Part model, mm, in its own coordinate system. Face numbers are marked on the shaded views. Coordinates: 2 decimals unless noted, no trailing zeros. Write each loop counter-clockwise with the first axis right and the second up, starting at its lowest first coordinate (ties: lowest second). Pieces come first, ordered by that corner, then holes. Notation, with made-up numbers: M 74.5,-3.75 L 114.5,-3.75 A16 ccw 114.5,10.25 Z; hole C -38,73 d10. An arc over 180 degrees is marked long. Use a Markdown table: item, result. Add a question column.
Q1. Slice it at B-B on y = 0. Write the cut outline in (x, z), then the cut area to 3 significant figures.
Q2. Slice it at D-D on z = 5.5. Write the cut outline in (x, y).
Q3. Wall check: L1, parallel to Y at x = -34, z = 3.5; L2, parallel to Y at x = -12.5, z = 5.25; L3, parallel to X at y = -29, z = 2. Give the ranges that are in metal, low to high. Write a range as from..to.
Q4. Mould opens along Y. For the marked faces 1, 2 and 3 say: released by +Y, released by -Y, zero draft, split by the parting line, or undercut.
Q5. Slice it at C-C on x = 50.5. Write the cut outline in (y, z).
Q6. Pin check, flat tips, straight feed: pin 1 Ø3 at (x, z) = (-56.5, 5.5) entering from +Y; pin 2 Ø3 at (y, z) = (-53, 3.5) entering from -X; pin 3 Ø5 at (x, z) = (25.5, 2) entering from +Y. Stop position of each tip, or through.
Q7. Slice it at A-A on x = 0. Write the cut outline in (y, z).
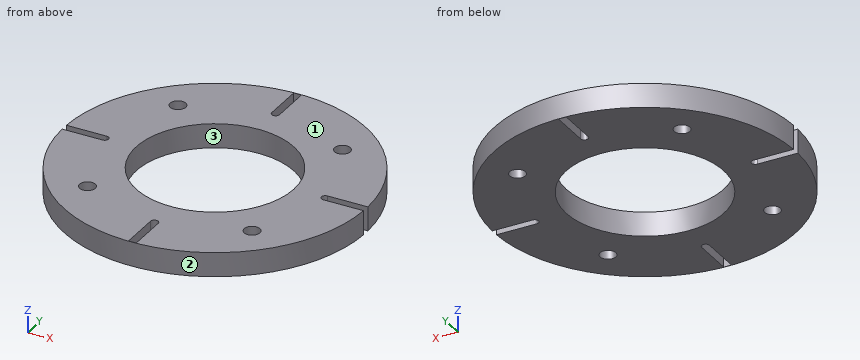
from build123d import *

# Parameters (mm, degrees)
IZIM1_R                     = 62.2
Y_KSEKLIK_EKSTR_ZYON1_DEPTH = 10
IZIM2_R                     = 32.5
KES_EKSTR_ZYON1_DEPTH       = 10
KES_EKSTR_ZYON2_DEPTH       = 10
IZIM5_R                     = 3.25
KES_EKSTR_ZYON3_DEPTH       = 10


with BuildPart() as part:
    # Çizim1 → Yükseklik-Ekstrüzyon1 (new body)
    with BuildSketch(Plane.XY):
        Circle(IZIM1_R)
    extrude(amount=Y_KSEKLIK_EKSTR_ZYON1_DEPTH)

    # Çizim2 → Kes-Ekstrüzyon1 (cut)
    with BuildSketch(Plane.XY.offset(10)):
        Circle(IZIM2_R)
    extrude(amount=-KES_EKSTR_ZYON1_DEPTH, mode=Mode.SUBTRACT)

    # Çizim4 → Kes-Ekstrüzyon2 (cut)
    with BuildSketch(Plane.XY.offset(10)):
        with BuildLine():
            Line((1.6, -62), (1.6, -45.5))
            ThreePointArc((1.6, -45.5), (0, -43.9), (-1.6, -45.5))
            Line((-1.6, -45.5), (-1.6, -62))
            Line((-1.6, -62), (1.6, -62))
        make_face()
        with BuildLine():
            Line((-1.6, 62), (-1.6, 45.5))
            ThreePointArc((-1.6, 45.5), (0, 43.9), (1.6, 45.5))
            Line((1.6, 45.5), (1.6, 62))
            Line((1.6, 62), (-1.6, 62))
        make_face()
        with BuildLine():
            Line((62.2, 1.6), (62.2, -1.6))
            Line((62.2, -1.6), (45.5, -1.6))
            ThreePointArc((45.5, -1.6), (43.9, 0), (45.5, 1.6))
            Line((45.5, 1.6), (62.2, 1.6))
        make_face()
        with BuildLine():
            Line((-62.2, -1.6), (-45.5, -1.6))
            ThreePointArc((-45.5, -1.6), (-43.9, 0), (-45.5, 1.6))
            Line((-45.5, 1.6), (-62.2, 1.6))
            Line((-62.2, 1.6), (-62.2, -1.6))
        make_face()
    extrude(amount=-KES_EKSTR_ZYON2_DEPTH, mode=Mode.SUBTRACT)

    # Çizim5 → Kes-Ekstrüzyon3 (cut)
    with BuildSketch(Plane(origin=(0, 0, 0), x_dir=(-1, 0, 0), z_dir=(0, 0, -1))):
        with Locations((-33.941125497, 33.941125497)):
            Circle(IZIM5_R)
        with Locations((33.941125497, 33.941125497)):
            Circle(IZIM5_R)
        with Locations((33.941125497, -33.941125497)):
            Circle(IZIM5_R)
        with Locations((-33.941125497, -33.941125497)):
            Circle(IZIM5_R)
    extrude(amount=-KES_EKSTR_ZYON3_DEPTH, mode=Mode.SUBTRACT)


solid = part.part
Recorded:
| question | item | result |
|---|---|---|
| 1 | outline | M -43.9,0 L -32.5,0 L -32.5,10 L -43.9,10 Z; M 32.5,0 L 43.9,0 L 43.9,10 L 32.5,10 Z |
| 1 | area | 228 mm² |
| 2 | outline | M -62.18,-1.6 A62.2 ccw 62.18,-1.6 L 45.5,-1.6 A1.6 cw 45.5,1.6 L 62.18,1.6 A62.2 ccw -62.18,1.6 L -45.5,1.6 A1.6 cw -45.5,-1.6 Z; hole C -33.94,-33.94 d6.5; hole C -33.94,33.94 d6.5; hole C 0,0 d65; hole M -1.6,-62 L 1.6,-62 L 1.6,-45.5 A1.6 ccw -1.6,-45.5 Z; hole M -1.6,45.5 A1.6 ccw 1.6,45.5 L 1.6,62 L -1.6,62 Z; hole C 33.94,-33.94 d6.5; hole C 33.94,33.94 d6.5 |
| 3 | L1 | -52.08..-37.19, -30.69..30.69, 37.19..52.08 |
| 3 | L2 | -60.93..-30, 30..60.93 |
| 3 | L3 | -55.03..-14.67, 14.67..55.03 |
| 4 | face 1 | zero draft |
| 4 | face 2 | released by -Y |
| 4 | face 3 | undercut |
| 5 | outline | M -36.31,0 L -1.6,0 L -1.6,10 L -36.31,10 Z; M 1.6,0 L 36.31,0 L 36.31,10 L 1.6,10 Z |
| 6 | pin 1 | y = 29.05 |
| 6 | pin 2 | x = -34.88 |
| 6 | pin 3 | y = 57.79 |
| 7 | outline | M -62.2,0 L -62,0 L -62,10 L -62.2,10 Z; M -43.9,0 L -32.5,0 L -32.5,10 L -43.9,10 Z; M 32.5,0 L 43.9,0 L 43.9,10 L 32.5,10 Z; M 62,0 L 62.2,0 L 62.2,10 L 62,10 Z |
